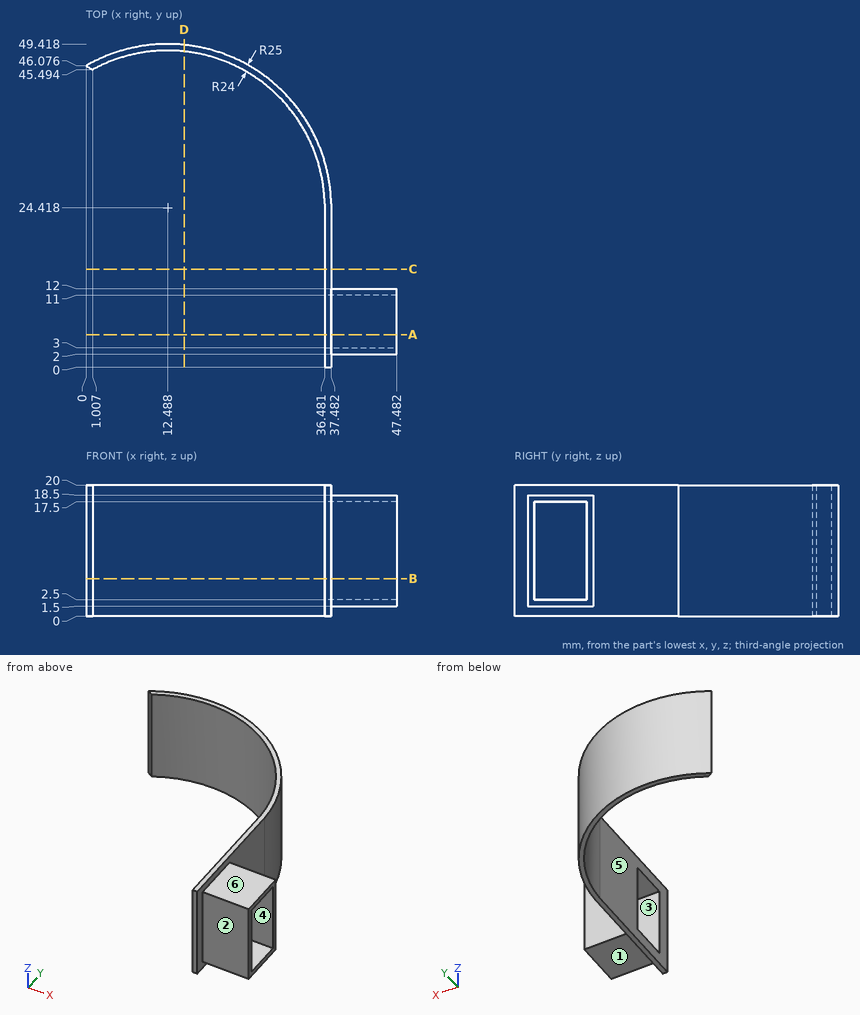
Answer from the drawing. Dimensions are ordinates in mm from the lowest x, y and z of the part. A direction names the side the tool comes from. Coordinates: 2 decimals unless noted, no trailing zeros. Write each loop counter-clockwise with the first axis right and the second up, starting at its lowest first coordinate (ties: lowest second). Pieces come first, ordered by that corner, then holes. Notation, with made-up numbers: M -9.75,54.25 L 10.25,54.25 A12 cw 10.25,67.25 Z; hole C 19.25,71.5 d10. An arc over 180 degrees is marked long. Put each result on its own line as item: value. Start each with the question number.
1. A cutting plane is placed at D-D on x = 15. Write down the section's boundary in (y, z), then the cut area to 3 significant figures.
2. Which of the six approach directions +Z, -Z, +X, -X, +Y, -Y give full straight-line access (tool end or side, diameter ignored) to the marked faces 4, 5 and 6?
3. Flat-ended cylindrical pins translate along their axes: P1, Ø4, axis at y = 5.5, z = 2.5, coming from the -X side; P2, Ø8, axis at x = 42, y = 9, coming from the -Z side; P3, Ø1, axis at x = 21.5, z = 4, coming from the -Y side. Find the tip coordinate at first contact, or state that the pin passes through.
4. A cutting plane is placed at C-C on y = 15. Write down the section's boundary in (x, z), then the cut area to 3 significant figures.
5. Consider line 1 (X direction, y = 14, z = 11.75); line 2 (Y direction, x = 43.5, z = 4.75); line 3 (Y direction, x = 41, z = 1.75). Determine where each line is inside the solid, lowest interval first. Write a range as from..to.
6. For a pull along Z with two mould halves and no side action, classify the marked faces 1, 2 and 3 as pulls with the +Z half, pulls with the -Z half, needs draft (parallel to the pull), parting line crosses it, or undercut.
7. A cutting plane is placed at A-A on y = 5. Write down the section's boundary in (x, z).
8. A cutting plane is placed at B-B on z = 5.75. Write down the section's boundary in (x, y) (1 decimal).
Resolved:
1. outline: M 48.29,0 L 49.29,0 L 49.29,20 L 48.29,20 Z
1. area: 20.1 mm2
2. face 4: +X, -X
2. face 5: +Z, -Z, -X, -Y
2. face 6: +Z, +X, +Y, -Y
3. P1: stops at x = 36.48
3. P2: stops at z = 1.5
3. P3: stops at y = 46.45
4. outline: M 36.48,0 L 37.48,0 L 37.48,20 L 36.48,20 Z
4. area: 20.0 mm2
5. line 1: x = 36.48..37.48
5. line 2: y = 2..3, 11..12
5. line 3: y = 2..12
6. face 1: pulls with the -Z half
6. face 2: needs draft
6. face 3: undercut
7. outline: M 36.48,0 L 37.48,0 L 37.48,1.5 L 47.48,1.5 L 47.48,2.5 L 36.48,2.5 Z; M 36.48,17.5 L 47.48,17.5 L 47.48,18.5 L 37.48,18.5 L 37.48,20 L 36.48,20 Z
8. outline: M 0,46.1 L 1,45.5 A24 cw 36.5,25 L 36.5,11 L 47.5,11 L 47.5,12 L 37.5,12 L 37.5,25 A25 ccw Z; M 36.5,0 L 37.5,0 L 37.5,2 L 47.5,2 L 47.5,3 L 36.5,3 Z
